Verification items for the finished model (mm, model axes). Give positions to 0.01 mm unless a question says otherwise; leave off trailing zeros. Loops run counter-clockwise (first coordinate to the right, second up) from the corner with the lowest first, then second, coordinate; pieces in that order, holes last. Notation, with made-up numbers: M 4.25,53 L 63.25,53 A31 cw 63.25,79 Z; hole C -8,67 d3. An arc over 180 degrees is marked long. Use a Markdown table: item, result.
from build123d import *

# Parameters (mm, degrees)
SKETCH1_R           = 1
BOSS_EXTRUDE1_DEPTH = 3


with BuildPart() as part:
    # Sketch1 → Boss-Extrude1 (new body)
    with BuildSketch(Plane.XY):
        with BuildLine():
            Line((0, 2), (60, 2))
            ThreePointArc((60, 2), (62, 0), (60, -2))
            Line((60, -2), (0, -2))
            ThreePointArc((0, -2), (-2, 0), (0, 2))
        make_face()
        Circle(SKETCH1_R, mode=Mode.SUBTRACT)
        with Locations((8, 0)):
            Circle(SKETCH1_R, mode=Mode.SUBTRACT)
        with Locations(Location((52, 0, 0), (0, 0, 180))):
            Circle(SKETCH1_R, mode=Mode.SUBTRACT)
        with Locations(Location((60, 0, 0), (0, 0, 180))):
            Circle(SKETCH1_R, mode=Mode.SUBTRACT)
    extrude(amount=BOSS_EXTRUDE1_DEPTH)


solid = part.part
(1) Material ranges on line 1 (Y direction, x = 52, z = 1.25); line 2 (X direction, y = -0.35, z = 1.35); line 3 (X direction, y = 0.75, z = 2.65), recorded low to high.
Results below:
| item | result |
|---|---|
| line 1 | -2 to -1, 1 to 2 |
| line 2 | -1.97 to -0.94, 0.94 to 7.06, 8.94 to 51.06, 52.94 to 59.06, 60.94 to 61.97 |
| line 3 | -1.85 to -0.66, 0.66 to 7.34, 8.66 to 51.34, 52.66 to 59.34, 60.66 to 61.85 |
(2) Cross-section at B-B on z = 1.8. Record the cut outline in (x, y).
Results below:
| item | result |
|---|---|
| outline | M 0,-2 L 60,-2 A2 ccw 60,2 L 0,2 A2 ccw Z; hole C 0,0 d2; hole C 8,0 d2; hole C 52,0 d2; hole C 60,0 d2 |
(3) Draft check along X on faces 1 (the cylindrical face through (62, 0, 1)), 2 (the cylindrical face through (-2, 0, 1)), 3 (the cylindrical face through (0, -1, 1)), 4 (the flat face through (30, -2, 1)). Enter one of: +X half, -X half, draft (parallel to the pull), parting line (faces both ways), or undercut.
Results below:
| item | result |
|---|---|
| face 1 | +X half |
| face 2 | -X half |
| face 3 | undercut |
| face 4 | draft |
(4) Cross-section at C-C on y = 0. Record the cut outline in (x, z), then the cut area to 3 significant figures.
Results below:
| item | result |
|---|---|
| outline | M -2,0 L -1,0 L -1,3 L -2,3 Z; M 1,0 L 7,0 L 7,3 L 1,3 Z; M 9,0 L 51,0 L 51,3 L 9,3 Z; M 53,0 L 59,0 L 59,3 L 53,3 Z; M 61,0 L 62,0 L 62,3 L 61,3 Z |
| area | 168 mm^2 |
(5) Cross-section at A-A on x = 8. Record the cut outline in (y, z).
Results below:
| item | result |
|---|---|
| outline | M -2,0 L -1,0 L -1,3 L -2,3 Z; M 1,0 L 2,0 L 2,3 L 1,3 Z |
